Geometry check sheet. Reference: drawing and pictorial views, mm from the part's lowest x, y, z. A direction names the side the tool comes from. Round coordinates to 2 decimals unless told otherwise and drop trailing zeros. Write each loop counter-clockwise with the first axis right and the second up, starting at its lowest first coordinate (ties: lowest second). Pieces come first, ordered by that corner, then holes. Notation, with made-up numbers: (37, 88) -> (41, 88) arc R25 ccw to (41, 119) -> close; hole circle Ø9 at (-8, 21). An arc over 180 degrees is marked (long way). Answer as a JSON object with one key per item and string values. Group by question number.
(1) Gauge pin test, flat ends, axial feed: pin 1 Ø14.5 at (x, z) = (22.5, 48) entering from -Y; pin 2 Ø14.5 at (x, z) = (27.5, 54) entering from +Y; pin 3 Ø23 at (x, y) = (19, 76.5) entering from -Z. Record the tip position at first contact, or that the pin passes through.
(2) Scan lines: L1, parallel to Y at x = 30, z = 44; L2, parallel to Y at x = 18.5, z = 46; L3, parallel to X at y = 23.8, z = 42.9. Record each from-to range of solid material in increasing order. Write a range as from..to.
(3) Sectioned sample at C-C on x = 9. Record the cut outline in (y, z), and give its area (3 significant figures).
(4) Sectioned sample at B-B on y = 21.5. Record the cut outline in (x, z), and give its area (3 significant figures).
(5) Sectioned sample at A-A on x = 30.3. Record the cut outline in (y, z).
(6) Draft check along Z on the marked faces 5, 6 and 7. Enter one of: released by +Z, released by -Z, zero draft, split by the parting line, or undercut.
(7) Set-up check for the marked faces 1, 2, 3 and 4: record each of +Z, -Z, +X, -X, +Y, -Y from which the full face is reachable in a straight line by a thin tool's end or side.
(8) Sectioned sample at D-D on y = 50. Record the cut outline in (x, z).
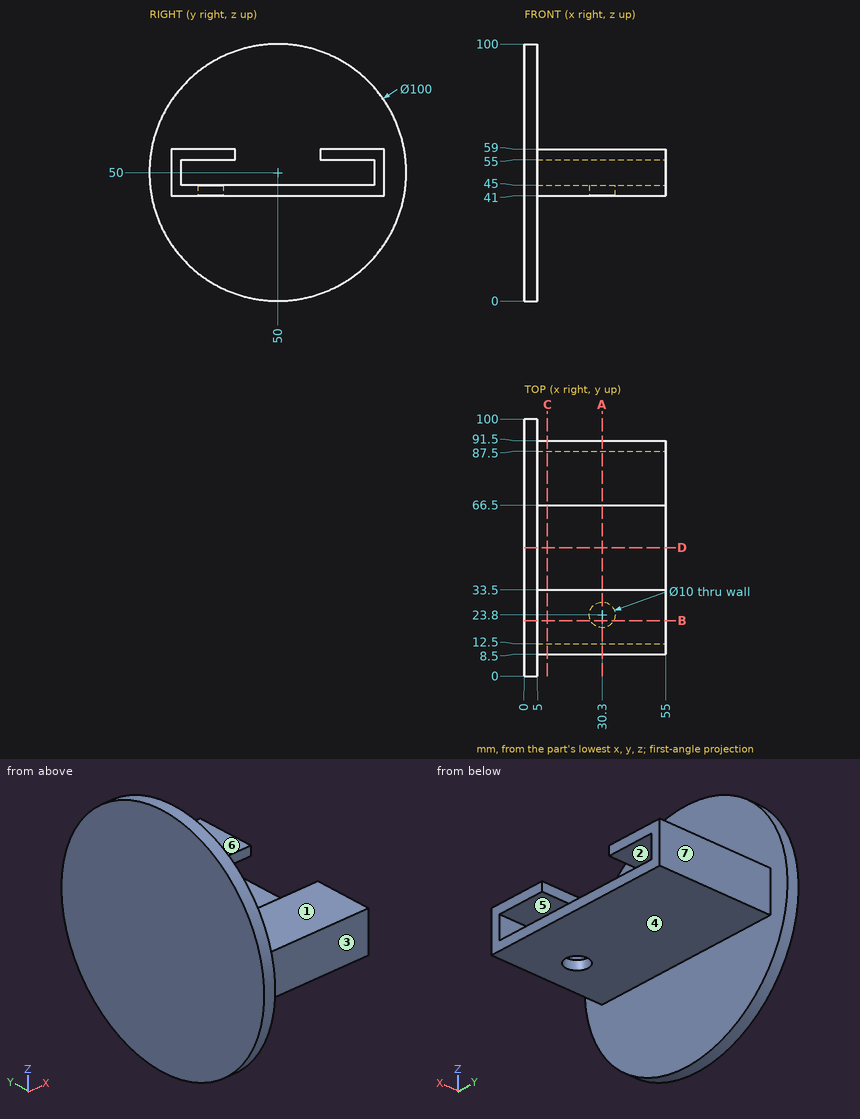
Computed values:
{
 "1": {"pin 1": "y = 8.5", "pin 2": "y = 91.5", "pin 3": "z = 41"},
 "2": {"L1": "8.5..18.81, 28.79..91.5", "L2": "8.5..12.5, 87.5..91.5", "L3": "0..25.3, 35.3..55"},
 "3": {"outline": "(8.5, 41) -> (91.5, 41) -> (91.5, 59) -> (66.5, 59) -> (66.5, 55) -> (87.5, 55) -> (87.5, 45) -> (12.5, 45) -> (12.5, 55) -> (33.5, 55) -> (33.5, 59) -> (8.5, 59) -> close", "area": "612 mm2"},
 "4": {"outline": "(0, 8.92) -> (5, 8.92) -> (5, 41) -> (25.86, 41) -> (25.86, 45) -> (5, 45) -> (5, 55) -> (55, 55) -> (55, 59) -> (5, 59) -> (5, 91.08) -> (0, 91.08) -> close; (34.74, 41) -> (55, 41) -> (55, 45) -> (34.74, 45) -> close", "area": "775 mm2"},
 "5": {"outline": "(8.5, 41) -> (18.8, 41) -> (18.8, 45) -> (12.5, 45) -> (12.5, 55) -> (33.5, 55) -> (33.5, 59) -> (8.5, 59) -> close; (28.8, 41) -> (91.5, 41) -> (91.5, 59) -> (66.5, 59) -> (66.5, 55) -> (87.5, 55) -> (87.5, 45) -> (28.8, 45) -> close"},
 "6": {"face 5": "undercut", "face 6": "released by +Z", "face 7": "zero draft"},
 "7": {"face 1": "+Z, +X, +Y, -Y", "face 2": "+X", "face 3": "+Z, -Z, +X, -Y", "face 4": "-Z, +X, +Y, -Y"},
 "8": {"outline": "(0, 0) -> (5, 0) -> (5, 41) -> (55, 41) -> (55, 45) -> (5, 45) -> (5, 100) -> (0, 100) -> close"}
}
